from build123d import *

# Parameters (mm, degrees)
SKETCH1_W                = 460
SKETCH1_H                = 250
BOSS_EXTRUDE1_DEPTH      = 16
SKETCH2_W                = 460
SKETCH2_H                = 169
CUT_EXTRUDE1_DEPTH       = 3
F_6_0_6_DIAMETER_HOLE1_D = 6
F_8_0MM_DOWEL_HOLE1_D    = 8
M8_TAPPED_HOLE1_D        = 6.8
M6_TAPPED_HOLE1_D        = 5
M5_TAPPED_HOLE1_D        = 4.2
CUT_EXTRUDE2_DEPTH       = 263.261320061
CHAMFER1_SIZE            = 5


with BuildPart() as part:
    # Sketch1 → Boss-Extrude1 (new body)
    with BuildSketch(Plane(origin=(0, 0, 0), x_dir=(1, 0, 0), z_dir=(0, 1, 0))):
        Rectangle(SKETCH1_W, SKETCH1_H)
    extrude(amount=BOSS_EXTRUDE1_DEPTH)

    # Sketch2 → Cut-Extrude1 (cut)
    with BuildSketch(Plane(origin=(0, 16, 0), x_dir=(1, 0, 0), z_dir=(0, 1, 0))):
        Rectangle(SKETCH2_W, SKETCH2_H)
    extrude(amount=-CUT_EXTRUDE1_DEPTH, mode=Mode.SUBTRACT)

    # Ø6.0 (6) Diameter Hole1 (through all)
    with Locations(Plane(origin=(0, 13, 0), x_dir=(1, 0, 0), z_dir=(0, 1, 0))):
        with Locations((0, 0)):
            Hole(F_6_0_6_DIAMETER_HOLE1_D / 2)

    # Ø8.0mm Dowel Hole1 (through all)
    with Locations(Plane(origin=(0, 13, 0), x_dir=(1, 0, 0), z_dir=(0, 1, 0))):
        with Locations((42, 12.5), (42, -12.5), (165.5, 56.5), (165.5, -56.5), (-218, 12.5), (-218, -12.5)):
            Hole(F_8_0MM_DOWEL_HOLE1_D / 2)

    # M8 Tapped Hole1 (through all)
    with Locations(Plane(origin=(0, 13, 0), x_dir=(1, 0, 0), z_dir=(0, 1, 0))):
        with Locations((42, 30), (42, -30), (143, 56.5), (188, 56.5), (188, -56.5), (143, -56.5), (-218, 30), (-218, -30)):
            Hole(M8_TAPPED_HOLE1_D / 2)

    # M6 Tapped Hole1 (through all)
    with Locations(Plane(origin=(0, 13, 0), x_dir=(1, 0, 0), z_dir=(0, 1, 0))):
        with Locations((-175, 73), (-115, 73), (-55, 73), (-175, -73), (-115, -73), (-55, -73)):
            Hole(M6_TAPPED_HOLE1_D / 2)

    # M5 Tapped Hole1 (through all)
    with Locations(Plane(origin=(0, 13, 0), x_dir=(1, 0, 0), z_dir=(0, 1, 0))):
        with Locations((-56.3, 29), (-56.3, -29), (-68.8, 29), (-68.8, -29), (-173.8, 29), (-173.8, -29), (-161.3, 29), (-161.3, -29)):
            Hole(M5_TAPPED_HOLE1_D / 2)

    # Sketch13 → Cut-Extrude2 (cut, through all)
    with BuildSketch(Plane(origin=(0, 16, 0), x_dir=(1, 0, 0), z_dir=(0, 1, 0))):
        with BuildLine():
            Line((-221.8, 105), (-221.8, 110))
            ThreePointArc((-221.8, 110), (-215, 116.8), (-208.2, 110))
            Line((-208.2, 110), (-208.2, 105))
            ThreePointArc((-208.2, 105), (-215, 98.2), (-221.8, 105))
        make_face()
        with BuildLine():
            Line((-6.8, 105), (-6.8, 110))
            ThreePointArc((-6.8, 110), (0, 116.8), (6.8, 110))
            Line((6.8, 110), (6.8, 105))
            ThreePointArc((6.8, 105), (0, 98.2), (-6.8, 105))
        make_face()
        with BuildLine():
            Line((208.2, 105), (208.2, 110))
            ThreePointArc((208.2, 110), (215, 116.8), (221.8, 110))
            Line((221.8, 110), (221.8, 105))
            ThreePointArc((221.8, 105), (215, 98.2), (208.2, 105))
        make_face()
        with BuildLine():
            Line((221.8, -105), (221.8, -110))
            ThreePointArc((221.8, -110), (215, -116.8), (208.2, -110))
            Line((208.2, -110), (208.2, -105))
            ThreePointArc((208.2, -105), (215, -98.2), (221.8, -105))
        make_face()
        with BuildLine():
            Line((6.8, -105), (6.8, -110))
            ThreePointArc((6.8, -110), (0, -116.8), (-6.8, -110))
            Line((-6.8, -110), (-6.8, -105))
            ThreePointArc((-6.8, -105), (0, -98.2), (6.8, -105))
        make_face()
        with BuildLine():
            Line((-208.2, -105), (-208.2, -110))
            ThreePointArc((-208.2, -110), (-215, -116.8), (-221.8, -110))
            Line((-221.8, -110), (-221.8, -105))
            ThreePointArc((-221.8, -105), (-215, -98.2), (-208.2, -105))
        make_face()
    extrude(amount=-CUT_EXTRUDE2_DEPTH, mode=Mode.SUBTRACT)

    # Chamfer1
    chamfer1_edges = [part.edges().sort_by_distance(p)[0] for p in [
        (230, 8, 125),
        (-230, 8, 125),
        (-230, 8, -125),
        (230, 8, -125),
    ]]
    chamfer(chamfer1_edges, length=CHAMFER1_SIZE)


solid = part.part
Geometry: final body of the model. Coordinates: model frame, mm. A direction names the side the tool comes from. Give positions to 0.01 mm unless a question says otherwise; leave off trailing zeros. Loops run counter-clockwise (first coordinate to the right, second up) from the corner with the lowest first, then second, coordinate; pieces in that order, holes last. Notation, with made-up numbers: M 65,-14.5 L 77,-14.5 A26 cw 77,13.5 Z; hole C -35.5,28 d2. An arc over 180 degrees is marked long. Put each result on its own line as item: value.
1) Cut plane A-A, the plane x = 20.5. Return the cut outline in (y, z).
Computed values:
outline: M 0,-125 L 16,-125 L 16,-84.5 L 13,-84.5 L 13,84.5 L 16,84.5 L 16,125 L 0,125 Z
2) Cut plane B-B, the plane y = 10.5. Give the number of separate pieces and of enclosed holes in the cut face, plus the area to 3 significant figures.
Computed values:
separate pieces: 1
enclosed holes: 35
area: 113,000 mm^2
3) Material intervals for L1, parallel to X at y = 10.25, z = 56.5; L2, parallel to Z at x = -68.8, y = 4; L3, parallel to X at y = 8.5, z = -13, sorted ascending. Write a range as from..to.
Computed values:
L1: x = -230..139.6, 146.4..161.5, 169.5..184.6, 191.4..230
L2: z = -125..-31.1, -26.9..26.9, 31.1..125
L3: x = -230..-221.97, -214.03..38.03, 45.97..230
4) Mould query, pull axis Z, two halves, no side actions, for faces 1 (the flat face through (-3, 8, -125)), 2 (the flat face through (-3, 8, 125)), 3 (the cylindrical face through (214.9, 8.1, -116.8)), 4 (the flat face through (-3, 0, -2)). Classes: released by +Z, released by -Z, zero draft, split by the parting line, or undercut.
Computed values:
face 1: released by -Z
face 2: released by +Z
face 3: undercut
face 4: zero draft
5) First-contact query: P1, Ø9, axis at x = 143, z = 56.5, coming from the +Y side. Flat tip, straight axial feed; report the tip coordinate or a pass-through.
Computed values:
P1: stops at y = 13
6) Reachability of faces 5 (the cylindrical face through (0.1, 8.1, -98.2)), 6 (the flat face through (-230, 6, 2)), 7 (the flat face through (-3, 13, -1)) from +Z, -Z, +X, -X, +Y, -Y: full face, straight path, thin tool, end or side. Return the list, or none.
Computed values:
face 5: +Y, -Y
face 6: +Z, -Z, -X, +Y, -Y
face 7: +X, -X, +Y
